Geometry check sheet. Reference: drawing and pictorial views, mm from the part's lowest x, y, z. A direction names the side the tool comes from. Give positions to 0.01 mm unless a question says otherwise; leave off trailing zeros. Loops run counter-clockwise (first coordinate to the right, second up) from the corner with the lowest first, then second, coordinate; pieces in that order, holes last. Notation, with made-up numbers: M -30,4 L -1,4 A23 cw -1,18 Z; hole C 35.25,20.5 d4. An arc over 180 degrees is marked long. One line per question, with ' | ' between items. Start each with the question number.
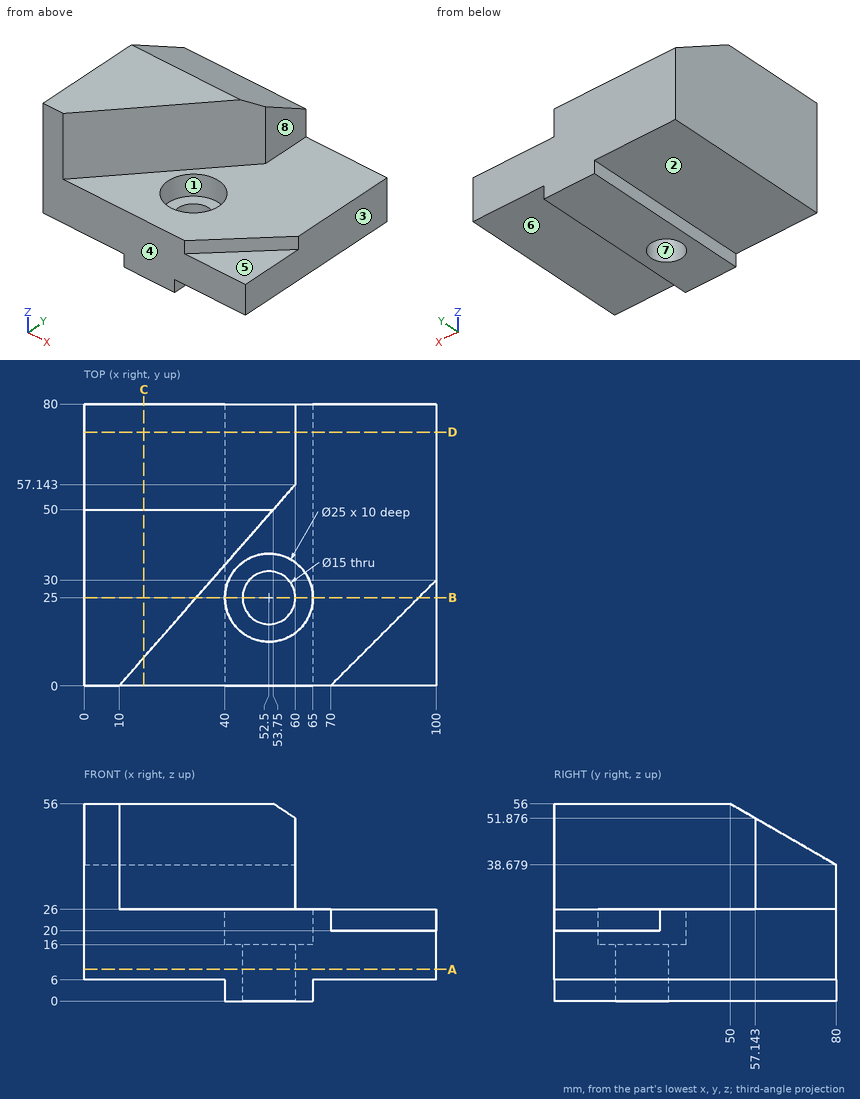
Q1. Material ranges on probe 1 along X at (y, z) = (25, 19.25); probe 2 along Y at (x, z) = (52.5, 8.5); probe 3 along Y at (x, z) = (52.5, 18.5), recorded low to high. Write a range as from..to.
Q2. Cross-section at A-A (z = 9). Record the cut outline in (x, y), and give its area (3 significant figures).
Q3. Depth check by flat-ended pin: P1, Ø24, axis at x = 52.5, y = 25, coming from the +Z side; P2, Ø20, axis at x = 57, y = 27, coming from the +Z side; P3, Ø10, axis at x = 61, y = 68, coming from the +Z side (1 decimal). Enter the tip coordinate at first touch or a pass-through.
Q4. Cross-section at C-C (x = 17). Record the cut outline in (y, z).
Q5. Cross-section at B-B (y = 25). Record the cut outline in (x, z) (1 decimal).
Q6. Draft check along X on the marked faces 6, 7 and 8. Enter one of: released by +X, released by -X, zero draft, split by the parting line, or undercut.
Q7. Access from +Z, -Z, +X, -X, +Y, -Y to the whole of each face (thin tool, end or side, straight path). Record for the marked faces 1, 2, 3, 4 and 5.
Q8. Cross-section at D-D (y = 72). Record the cut outline in (x, z), and give its area (3 significant figures).
Solved:
1) probe 1: x = 0..40, 65..100 | probe 2: y = 0..17.5, 32.5..80 | probe 3: y = 0..12.5, 37.5..80
2) outline: M 0,0 L 100,0 L 100,80 L 0,80 Z; hole C 52.5,25 d15 | area: 7,820 mm²
3) P1: stops at z = 16 | P2: stops at z = 26 | P3: stops at z = 48.4
4) outline: M 0,6 L 80,6 L 80,38.68 L 50,56 L 8,56 L 8,26 L 0,26 Z
5) outline: M 0,6 L 40,6 L 40,0 L 45,0 L 45,16 L 40,16 L 40,26 L 31.9,26 L 31.9,56 L 0,56 Z; M 60,0 L 65,0 L 65,6 L 100,6 L 100,20 L 95,20 L 95,26 L 65,26 L 65,16 L 60,16 Z
6) face 6: zero draft | face 7: undercut | face 8: released by +X
7) face 1: +Z | face 2: -Z, -X, +Y, -Y | face 3: +Z, -Z, +X, +Y, -Y | face 4: +Z, -Z, +X, -X, -Y | face 5: +Z, +X, -Y
8) outline: M 0,6 L 40,6 L 40,0 L 65,0 L 65,6 L 100,6 L 100,26 L 60,26 L 60,43.3 L 0,43.3 Z | area: 3,190 mm²
